from build123d import *

# Parameters (mm, degrees)
SKETCH1_W           = 100
SKETCH1_H           = 60
SKETCH1_R           = 12
BOSS_EXTRUDE1_DEPTH = 7
SKETCH4_R           = 8.075
CUT_EXTRUDE1_DEPTH  = 3
SKETCH5_R           = 3.5
CUT_EXTRUDE2_DEPTH  = 5
EXTRUDE_THIN1_START = 2
SKETCH6_R           = 10.075
SKETCH6_R_2         = 8.075
EXTRUDE_THIN1_DEPTH = 2
CHAMFER1_SIZE       = 2
SKETCH7_R           = 2.15
CUT_EXTRUDE3_DEPTH  = 85.654134571
FILLET1_R           = 5
CUT_EXTRUDE4_DEPTH  = 3
SKETCH9_R           = 16.1
CUT_EXTRUDE5_DEPTH  = 4
BOSS_EXTRUDE2_START = 3
SKETCH10_R          = 18
SKETCH10_R_2        = 16.1
BOSS_EXTRUDE2_DEPTH = 3
CHAMFER2_SIZE2      = 3
CHAMFER2_SIZE       = 1.732050808
SKETCH11_W          = 22.3
SKETCH11_H          = 60
SKETCH11_R          = 4.9
BOSS_EXTRUDE3_DEPTH = 7
FILLET2_R           = 5
SKETCH12_R          = 9
CUT_EXTRUDE6_DEPTH  = 4
SKETCH15_R          = 1.65
CUT_EXTRUDE7_DEPTH  = 10


with BuildPart() as part:
    # Sketch1 → Boss-Extrude1 (new body)
    with BuildSketch(Plane.XY):
        with Locations((-28.85, 0)):
            Rectangle(SKETCH1_W, SKETCH1_H)
        with Locations((-10, 0)):
            Circle(SKETCH1_R, mode=Mode.SUBTRACT)
        with BuildLine():
            Line((3.5, 13.85), (7.5, 13.85))
            ThreePointArc((7.5, 13.85), (9.15, 15.5), (7.5, 17.15))
            Line((7.5, 17.15), (3.5, 17.15))
            ThreePointArc((3.5, 17.15), (1.85, 15.5), (3.5, 13.85))
        make_face(mode=Mode.SUBTRACT)
        with BuildLine():
            Line((-27.5, 17.15), (-23.5, 17.15))
            ThreePointArc((-23.5, 17.15), (-21.85, 15.5), (-23.5, 13.85))
            Line((-23.5, 13.85), (-27.5, 13.85))
            ThreePointArc((-27.5, 13.85), (-29.15, 15.5), (-27.5, 17.15))
        make_face(mode=Mode.SUBTRACT)
        with BuildLine():
            Line((3.5, -17.15), (7.5, -17.15))
            ThreePointArc((7.5, -17.15), (9.15, -15.5), (7.5, -13.85))
            Line((7.5, -13.85), (3.5, -13.85))
            ThreePointArc((3.5, -13.85), (1.85, -15.5), (3.5, -17.15))
        make_face(mode=Mode.SUBTRACT)
        with BuildLine():
            Line((-27.5, -17.15), (-23.5, -17.15))
            ThreePointArc((-23.5, -17.15), (-21.85, -15.5), (-23.5, -13.85))
            Line((-23.5, -13.85), (-27.5, -13.85))
            ThreePointArc((-27.5, -13.85), (-29.15, -15.5), (-27.5, -17.15))
        make_face(mode=Mode.SUBTRACT)
    extrude(amount=BOSS_EXTRUDE1_DEPTH)

    # Sketch4 → Cut-Extrude1 (cut)
    with BuildSketch(Plane.XY.offset(7)):
        with Locations((-47.5, 0)):
            Circle(SKETCH4_R)
    extrude(amount=-CUT_EXTRUDE1_DEPTH, mode=Mode.SUBTRACT)

    # Sketch5 → Cut-Extrude2 (cut)
    with BuildSketch(Plane.XY.offset(4)):
        with Locations((-47.5, 0)):
            Circle(SKETCH5_R)
    extrude(amount=-CUT_EXTRUDE2_DEPTH, mode=Mode.SUBTRACT)

    # Sketch6 → Extrude-Thin1 (add)
    with BuildSketch(Plane.XY.offset(7).offset(EXTRUDE_THIN1_START)):
        with Locations((-47.5, 0)):
            Circle(SKETCH6_R)
        with Locations((-47.5, 0)):
            Circle(SKETCH6_R_2, mode=Mode.SUBTRACT)
    extrude(amount=-EXTRUDE_THIN1_DEPTH)

    # Chamfer1
    chamfer1_edges = [part.edges().sort_by_distance(p)[0] for p in [
        (-57.575, 0, 7),
    ]]
    chamfer(chamfer1_edges, length=CHAMFER1_SIZE - 0.0001)  # a hair under: the kernel refuses the full size

    # Sketch7 → Cut-Extrude3 (cut, through all)
    with BuildSketch(Plane.XY.offset(7)):
        with Locations((-68.85, 25)):
            Circle(SKETCH7_R)
        with Locations((-28.85, 25)):
            Circle(SKETCH7_R)
        with Locations((11.15, 25)):
            Circle(SKETCH7_R)
        with Locations((11.15, -25)):
            Circle(SKETCH7_R)
        with Locations((-28.85, -25)):
            Circle(SKETCH7_R)
        with Locations((-68.85, -25)):
            Circle(SKETCH7_R)
    extrude(amount=-CUT_EXTRUDE3_DEPTH, mode=Mode.SUBTRACT)

    # Fillet1
    fillet1_edges = [part.edges().sort_by_distance(p)[0] for p in [
        (21.15, -30, 3.5),
        (-78.85, -30, 3.5),
        (-78.85, 30, 3.5),
        (21.15, 30, 3.5),
    ]]
    fillet(fillet1_edges, radius=FILLET1_R)

    # Sketch8 → Cut-Extrude4 (cut)
    with BuildSketch(Plane(origin=(0, 0, 0), x_dir=(-1, 0, 0), z_dir=(0, 0, -1))):
        Polygon((-9.273611625, 28.25), (-13.026388375, 28.25), (-14.90277675, 25), (-13.026388375, 21.75), (-9.273611625, 21.75), (-7.39722325, 25), align=None)
        Polygon((26.973611625, 21.75), (30.726388375, 21.75), (32.60277675, 25), (30.726388375, 28.25), (26.973611625, 28.25), (25.09722325, 25), align=None)
        Polygon((70.726388375, 21.75), (72.60277675, 25), (70.726388375, 28.25), (66.973611625, 28.25), (65.09722325, 25), (66.973611625, 21.75), align=None)
        Polygon((66.973611625, -28.25), (70.726388375, -28.25), (72.60277675, -25), (70.726388375, -21.75), (66.973611625, -21.75), (65.09722325, -25), align=None)
        Polygon((32.60277675, -25), (30.726388375, -21.75), (26.973611625, -21.75), (25.09722325, -25), (26.973611625, -28.25), (30.726388375, -28.25), align=None)
        Polygon((-7.39722325, -25), (-9.273611625, -21.75), (-13.026388375, -21.75), (-14.90277675, -25), (-13.026388375, -28.25), (-9.273611625, -28.25), align=None)
    extrude(amount=-CUT_EXTRUDE4_DEPTH, mode=Mode.SUBTRACT)

    # Sketch9 → Cut-Extrude5 (cut)
    with BuildSketch(Plane.XY.offset(7)):
        with Locations((-10, 0)):
            Circle(SKETCH9_R)
    extrude(amount=-CUT_EXTRUDE5_DEPTH, mode=Mode.SUBTRACT)

    # Sketch10 → Boss-Extrude2 (add)
    with BuildSketch(Plane.XY.offset(7).offset(BOSS_EXTRUDE2_START)):
        with Locations((-10, 0)):
            Circle(SKETCH10_R)
        with Locations((-10, 0)):
            Circle(SKETCH10_R_2, mode=Mode.SUBTRACT)
    extrude(amount=-BOSS_EXTRUDE2_DEPTH)

    # Chamfer2
    chamfer2_edges = [part.edges().sort_by_distance(p)[0] for p in [
        (-28, 0, 10),
    ]]
    chamfer2_side = [part.faces().sort_by_distance(p)[0] for p in [
        (-27.965358984, 0, 10),
    ]]
    chamfer(chamfer2_edges, length=CHAMFER2_SIZE - 0.0001, length2=CHAMFER2_SIZE2 - 0.0001, reference=chamfer2_side[0])  # a hair under: the kernel refuses the full size

    # Sketch11 → Boss-Extrude3 (add)
    with BuildSketch(Plane(origin=(0, 0, 0), x_dir=(-1, 0, 0), z_dir=(0, 0, -1))):
        with Locations((85, 0)):
            Rectangle(SKETCH11_W, SKETCH11_H)
        with Locations((85, 0)):
            Circle(SKETCH11_R, mode=Mode.SUBTRACT)
    extrude(amount=-BOSS_EXTRUDE3_DEPTH)

    # Fillet2
    fillet2_edges = [part.edges().sort_by_distance(p)[0] for p in [
        (-96.15, 30, 3.5),
        (-96.15, -30, 3.5),
    ]]
    fillet(fillet2_edges, radius=FILLET2_R)

    # Sketch12 → Cut-Extrude6 (cut)
    with BuildSketch(Plane.XY.offset(7)):
        with Locations((-85, 0)):
            Circle(SKETCH12_R)
    extrude(amount=-CUT_EXTRUDE6_DEPTH, mode=Mode.SUBTRACT)

    # Sketch15 → Cut-Extrude7 (cut)
    with BuildSketch(Plane(origin=(0, 0, 0), x_dir=(-1, 0, 0), z_dir=(0, 0, -1))):
        with Locations((85, 18.61)):
            Circle(SKETCH15_R)
        with Locations((85, -18.61)):
            Circle(SKETCH15_R)
        with Locations((66.39, 0)):
            Circle(SKETCH15_R)
    extrude(amount=-CUT_EXTRUDE7_DEPTH, mode=Mode.SUBTRACT)


solid = part.part
Here's how the part is built. I have some questions about the finished solid (model axes, mm). A direction names the side the tool comes from. Give positions to 0.01 mm unless a question says otherwise; leave off trailing zeros. Use a Markdown table: item, result. Add a question column.
Item 1: For faces 5 (the face through (11, 28.25, 1)), 6 (the face through (-81, -4, 3)), 7 (the face through (6, -13.85, 3)), which set-ups out of +Z, -Z, +X, -X, +Y, -Y let a thin tool reach every point of the face, with its end or its side?
Item 2: Imagine slicing it at B-B on y = 0. Give the number of separate pieces and of enclosed holes in the cut face, plus the area to 3 significant figures.
Item 3: Will these pins go through, and if not, where does the flat tip stop? pin 1 (3 mm diameter, centred on x = 12, y = 24.5, fed in from -Z); pin 2 (20 mm diameter, centred on x = -85, y = 0, fed in from +Z); pin 3 (14.5 mm diameter, centred on x = -47.5, y = 0, fed in from +Z).
Item 4: I need wall thicknesses on line 1 (Y direction, x = -68.85, z = 4.25); line 2 (X direction, y = -2.5, z = 3.5); line 3 (X direction, y = -14, z = 6.5). Which ranges of each line are inside material? Lowest first, please.
Item 5: If we mould it in two halves opening along X, with no side actions, what happens to faces 1 (the face through (-94.65, 28.57, 3.55)), 2 (the face through (19.65, -28.57, 3.55)), 3 (the face through (-37, 30, 3)), 4 (the face through (-29, -28.25, 1))? For each: pulls with the +X half, pulls with the -X half, needs draft (parallel to the pull), parting line crosses it, or undercut.
Data:
| question | item | result |
|---|---|---|
| 1 | face 5 | -Z |
| 1 | face 6 | +Z |
| 1 | face 7 | +Z, -Z |
| 2 | separate pieces | 5 |
| 2 | enclosed holes | 0 |
| 2 | area | 438 mm² |
| 3 | pin 1 | stops at z = 3 |
| 3 | pin 2 | stops at z = 7 |
| 3 | pin 3 | stops at z = 4 |
| 4 | line 1 | y = -30 to -27.15, -22.85 to 22.85, 27.15 to 30 |
| 4 | line 2 | x = -96.15 to -93.65, -76.35 to -49.95, -45.05 to -25.9, 5.9 to 21.15 |
| 4 | line 3 | x = -96.15 to -28.19, -22.81 to -17.95, -2.05 to 2.81, 8.19 to 21.15 |
| 5 | face 1 | pulls with the -X half |
| 5 | face 2 | pulls with the +X half |
| 5 | face 3 | needs draft |
| 5 | face 4 | undercut |
